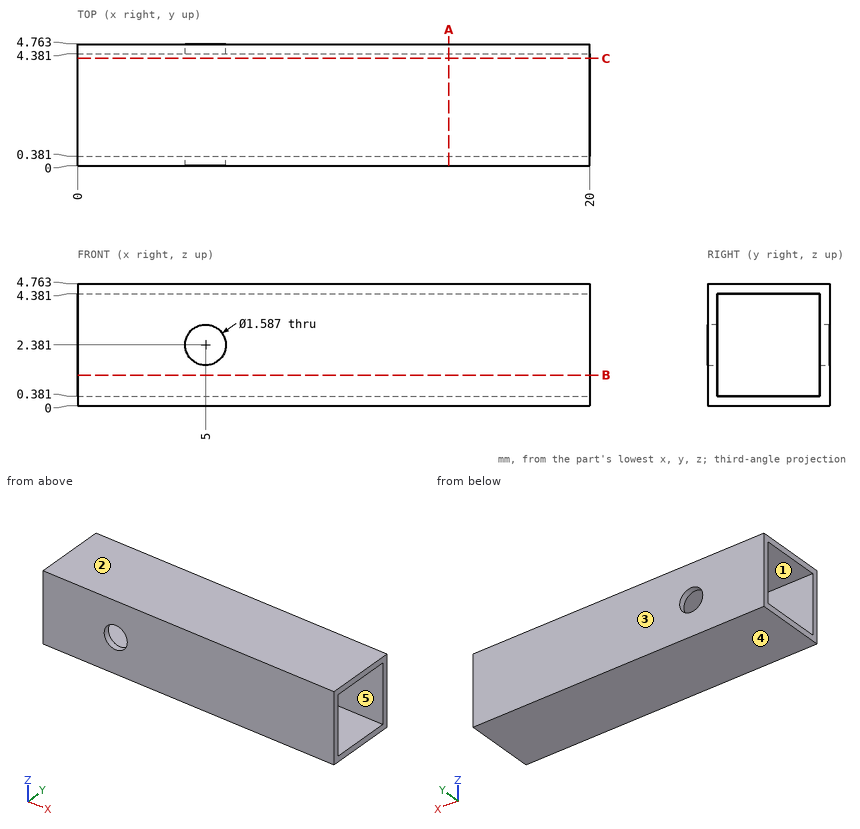
Part print with two shaded views. Sizes in mm from the minimum x, y, z corner. A direction names the side the tool comes from. Round coordinates to 2 decimals unless told otherwise and drop trailing zeros. Loops run counter-clockwise (first coordinate to the right, second up) from the corner with the lowest first, then second, coordinate; pieces in that order, holes last. Notation, with made-up numbers: (-40, -13.5) - (17, -13.5) arc R11 ccw to (17, -4.5) - close; hole circle Ø9 at (51.5, 83.5). An arc over 180 degrees is marked (long way). Answer as a JSON object with one key per item and string values.
Item 1: Band-saw the part on A-A on x = 14.5. List the corners of the cut face in (y, z).
Output:
{"outline": "(0, 0) - (4.76, 0) - (4.76, 4.76) - (0, 4.76) - close; hole (0.38, 0.38) - (4.38, 0.38) - (4.38, 4.38) - (0.38, 4.38) - close"}
Item 2: Band-saw the part on B-B on z = 1.2. List the corners of the cut face in (x, y).
Output:
{"outline": "(0, 0) - (20, 0) - (20, 0.38) - (0, 0.38) - close; (0, 4.38) - (20, 4.38) - (20, 4.76) - (0, 4.76) - close"}
Item 3: Pin check, flat tip, straight feed: pin 1 (1 mm diameter, centred on x = 10, z = 2.5, fed in from -Y). Stop position of the tip, or through.
Output:
{"pin 1": "y = 0"}
Item 4: Tool access for the marked faces 1 and 2: list every direction of +Z, -Z, +X, -X, +Y, -Y with a clear straight run to the whole face (end or side of a thin tool).
Output:
{"face 1": "+X, -X", "face 2": "+Z, +X, -X, +Y, -Y"}
Item 5: Wall check: L1, parallel to Y at x = 16.25, z = 3.9. Give the ranges that are in metal, low to high.
Output:
{"L1": "0 to 0.38, 4.38 to 4.76"}
Item 6: Pull direction Z, two halves, no side cores. Call the marked faces 3, 4 and 5: pulls with the +Z half, pulls with the -Z half, needs draft (parallel to the pull), parting line crosses it, or undercut.
Output:
{"face 3": "needs draft", "face 4": "pulls with the -Z half", "face 5": "undercut"}
